Autodesk Inventor part; units mm, degrees
ref_plane "YZ Plane" through (0, 0, 0) normal (1, 0, 0) x (0, 1, 0)
ref_plane "XZ Plane" through (0, 0, 0) normal (0, 1, 0) x (-1, 0, 0)
ref_plane "XY Plane" through (0, 0, 0) normal (0, 0, 1) x (1, 0, 0)
sketch "Sketch1" plane through (0, 0, 0) normal (0, 1, 0) x (-1, 0, 0)
  circle A0 centre (0, 0) radius 3
  dimension "d0" = 6
extrude "Extrusion1" add sketch "Sketch1" along normal blind 2.4
sketch "Sketch2" plane through (0, 2.4, 0) normal (0, 1, 0) x (1, 0, 0)
  line L0 (-1.55, 0.25) -> (1.55, 0.25)
  line L1 (1.55, 0.25) -> (1.55, -0.25)
  line L2 (1.55, -0.25) -> (-1.55, -0.25)
  line L3 (-1.55, -0.25) -> (-1.55, 0.25)
  line L4 (-0.25, -1.55) -> (0.25, -1.55)
  line L5 (0.25, -1.55) -> (0.25, 1.55)
  line L6 (0.25, 1.55) -> (-0.25, 1.55)
  line L7 (-0.25, 1.55) -> (-0.25, -1.55)
  point P0 (0, 0)
  dimension "d5" = 3.1
  dimension "d6" = 0.5
  dimension "d9" = 0.5
  dimension "d10" = 3.1
extrude "Extrusion2" cut sketch "Sketch2" against normal blind 1
fillet "Fillet1" radius 1 1 edges at (3, 2.4, 0)
sketch "Sketch3" plane through (0, 0, 0) normal (0, -1, 0) x (1, 0, 0)
  circle A0 centre (0, 0) radius 1.5
  dimension "d14" = 3
extrude "Extrusion3" add sketch "Sketch3" along normal blind 20
thread "Thread1"
properties part number "m3 20mm screw"
The listing builds one solid part. Answer for the finished solid, in the listing's coordinates (mm). A direction names the side the tool comes from. Round coordinates to 2 decimals unless told otherwise and drop trailing zeros. Write each loop counter-clockwise with the first axis right and the second up, starting at its lowest first coordinate (ties: lowest second). Pieces come first, ordered by that corner, then holes. Notation, with made-up numbers: (-35.5, 65.5) - (21.5, 65.5) arc R32 ccw to (21.5, 92.5) - close; hole circle Ø2 at (18, 72.25). An arc over 180 degrees is marked (long way). Use one line per item in the form item = value. Start each with the question number.
Item 1: A cutting plane is placed at C-C (y = -13.5). Write down the section's boundary in (x, z).
Item 2: Find the intervals of material crossed by line 1 (Y direction, x = 0.55, z = -1.75); line 2 (X direction, y = -18.5, z = -1); line 3 (Z direction, x = 1.35, y = -16.25), in increasing order. Write a range as [from, to].
Item 3: A tool of negligible diameter and unlimited length cuts with its end or side. For faces 4 (the flat face through (-1.3, 0, -1.3)), 5 (the flat face through (-0.4, 2.4, -0.4)), 6 (the flat face through (-1, 2, -0.25)), from which of +Z, -Z, +X, -X, +Y, -Y can it reach the whole face along a straight path? Write none if from no direction.
Item 4: A cutting plane is placed at B-B (x = 0). Write down the section's boundary in (y, z), plus the area to 3 significant figures.
Item 5: Flat-ended cylindrical pins translate along their axes: pin 1 Ø1.5 at (y, z) = (-1.5, 1.5) entering from +X; pin 2 Ø3 at (x, y) = (0, -6.5) entering from +Z; pin 3 Ø1.1 at (x, y) = (-1, 1.5) entering from +Z. Find the tip coordinate at first contact, or state that the pin passes through.
Item 6: A cutting plane is placed at A-A (z = 0). Write down the section's boundary in (x, y).
Item 7: Determine the mould class of faces 1 (the flat face through (1, 2, 0.25)), 2 (the flat face through (0, -20, 0)), 3 (the cylindrical face through (-1.5, -9.86, -0.07)) for opening direction X: +X half, -X half, draft (parallel to the pull), parting line (faces both ways), or undercut.
The answers:
q1.outline = circle Ø3 at (0, 0)
q2.line_1 = [0, 2.4]
q2.line_2 = [-1.12, 1.12]
q2.line_3 = [-0.65, 0.65]
q3.face_4 = -Y
q3.face_5 = +Z, -Z, +X, -X, +Y
q3.face_6 = +Y
q4.outline = (-20, -1.5) - (0, -1.5) - (0, -3) - (1.4, -3) arc R1 ccw to (2.4, -2) - (2.4, -1.55) - (1.4, -1.55) - (1.4, 1.55) - (2.4, 1.55) - (2.4, 2) arc R1 ccw to (1.4, 3) - (0, 3) - (0, 1.5) - (-20, 1.5) - close
q4.area = 70.9 mm^2
q5.pin_1 = 1.3
q5.pin_2 = 1.5
q5.pin_3 = 2.96
q6.outline = (-3, 0) - (-1.5, 0) - (-1.5, -20) - (1.5, -20) - (1.5, 0) - (3, 0) - (3, 1.4) arc R1 ccw to (2, 2.4) - (1.55, 2.4) - (1.55, 1.4) - (-1.55, 1.4) - (-1.55, 2.4) - (-2, 2.4) arc R1 ccw to (-3, 1.4) - close
q7.face_1 = undercut
q7.face_2 = draft
q7.face_3 = parting line
